The model under review builds one solid part; all positions refer to its coordinate system, in mm. A direction names the side the tool comes from. Coordinates: 2 decimals unless noted, no trailing zeros. Loops run counter-clockwise (first coordinate to the right, second up) from the corner with the lowest first, then second, coordinate; pieces in that order, holes last. Notation, with made-up numbers: M -36.75,1.5 L 18.25,1.5 A12 ccw 18.25,20.5 Z; hole C 70,22.25 d7. An arc over 180 degrees is marked long. Return JSON: item names as keys, results as strings.
```python
from build123d import *

# Parameters (mm, degrees)
SKETCH_1_W          = 220
SKETCH_1_H          = 180
EXTRUDE_1_DEPTH     = 395
SKETCH_17_W         = 46
SKETCH_17_H         = 45
CUT_EXTRUDE_2_DEPTH = 2
SKETCH_19_W         = 224
SKETCH_19_H         = 184
EXTRUDE_13_DEPTH    = 2
SKETCH_20_W         = 60
SKETCH_20_H         = 18
CUT_EXTRUDE_4_DEPTH = 65
SKETCH_21_W         = 144
SKETCH_21_H         = 332
CUT_EXTRUDE_5_DEPTH = 2
SKETCH_22_R         = 2.5
CUT_EXTRUDE_6_DEPTH = 10
SKETCH_23_R         = 11
SKETCH_23_R_2       = 2.25
SKETCH_23_R_3       = 1.5
CUT_EXTRUDE_7_DEPTH = 2
SKETCH_24_R         = 2
SKETCH_24_R_2       = 2.5
CUT_EXTRUDE_8_DEPTH = 3
CUT_EXTRUDE_9_DEPTH = 491.824815999
HOLE_WIZARD_M6_1_D  = 5


with BuildPart() as part:
    # 草图1 → 凸台-拉伸1 (new body)
    with BuildSketch(Plane(origin=(0, 0, 0), x_dir=(1, 0, 0), z_dir=(0, 1, 0))):
        Polygon((222, 2), (222, -182), (173, -182), (47, -182), (-2, -182), (-2, 2), align=None)
        with Locations((110, -90)):
            Rectangle(SKETCH_1_W, SKETCH_1_H, mode=Mode.SUBTRACT)
    extrude(amount=EXTRUDE_1_DEPTH)

    # 草图17 → 切除-拉伸2 (cut)
    with BuildSketch(Plane.XY.offset(182)):
        with Locations((23, 22.5)):
            Rectangle(SKETCH_17_W, SKETCH_17_H)
        with Locations((197, 22.5)):
            Rectangle(SKETCH_17_W, SKETCH_17_H)
    extrude(amount=-CUT_EXTRUDE_2_DEPTH, mode=Mode.SUBTRACT)

    # 草图19 → 凸台-拉伸13 (add)
    with BuildSketch(Plane(origin=(0, 395, 0), x_dir=(1, 0, 0), z_dir=(0, 1, 0))):
        with Locations((110, -90)):
            Rectangle(SKETCH_19_W, SKETCH_19_H)
    extrude(amount=EXTRUDE_13_DEPTH)

    # 草图20 → 切除-拉伸4 (cut)
    with BuildSketch(Plane.XY.offset(182)):
        with Locations((110, 390)):
            Rectangle(SKETCH_20_W, SKETCH_20_H)
    extrude(amount=-CUT_EXTRUDE_4_DEPTH, mode=Mode.SUBTRACT)

    # 草图21 → 切除-拉伸5 (cut)
    with BuildSketch(Plane(origin=(222, 0, 0), x_dir=(0, 0, -1), z_dir=(1, 0, 0))):
        with Locations((-90, 211)):
            Rectangle(SKETCH_21_W, SKETCH_21_H)
    extrude(amount=-CUT_EXTRUDE_5_DEPTH, mode=Mode.SUBTRACT)

    # 草图22 → 切除-拉伸6 (cut)
    with BuildSketch(Plane(origin=(0, 397, 0), x_dir=(1, 0, 0), z_dir=(0, 1, 0))):
        with Locations(Location((77.7, -25.2, 0), (0, 0, 270))):
            Circle(SKETCH_22_R)
        with Locations(Location((77.7, -89.8, 0), (0, 0, 270))):
            Circle(SKETCH_22_R)
        with Locations(Location((142.3, -89.8, 0), (0, 0, 270))):
            Circle(SKETCH_22_R)
        with Locations(Location((142.3, -25.2, 0), (0, 0, 270))):
            Circle(SKETCH_22_R)
        Polygon((74, -57.5), (74, -81.5), (146, -81.5), (146, -33.5), (74, -33.5), align=None)
    extrude(amount=-CUT_EXTRUDE_6_DEPTH, mode=Mode.SUBTRACT)

    # 草图23 → 切除-拉伸7 (cut)
    with BuildSketch(Plane(origin=(0, 0, -2), x_dir=(-1, 0, 0), z_dir=(0, 0, -1))):
        with Locations((-183.5, 217.109875683)):
            Circle(SKETCH_23_R)
        with Locations((-203.5, 88.459875683)):
            Circle(SKETCH_23_R_2)
        with Locations((-163.5, 88.459875683)):
            Circle(SKETCH_23_R_2)
        with Locations((-183.5, 180.109875683)):
            Circle(SKETCH_23_R)
        with Locations((-183.5, 254.109875683)):
            Circle(SKETCH_23_R)
        with Locations((-171.8, 147.859875683)):
            Circle(SKETCH_23_R_3)
        with Locations(Location((-195.2, 147.859875683, 0), (0, 0, 180))):
            Circle(SKETCH_23_R_3)
        Polygon((-183.5, 111.959875683), (-197.25, 111.959875683), (-197.25, 64.959875683), (-169.75, 64.959875683), (-169.75, 111.959875683), align=None)
        Polygon((-183.5, 151.609875683), (-175, 151.609875683), (-175.5, 143.109875683), (-183.5, 143.109875683), (-191.5, 143.109875683), (-192, 151.609875683), align=None)
    extrude(amount=-CUT_EXTRUDE_7_DEPTH, mode=Mode.SUBTRACT)

    # 草图24 → 切除-拉伸8 (cut)
    with BuildSketch(Plane(origin=(222, 0, 0), x_dir=(0, 0, -1), z_dir=(1, 0, 0))):
        with Locations((-169.5, 362)):
            Circle(SKETCH_24_R)
        with Locations((-169.5, 347)):
            Circle(SKETCH_24_R)
        with Locations(Location((-169.5, 75, 0), (0, 0, 180))):
            Circle(SKETCH_24_R)
        with Locations(Location((-169.5, 60, 0), (0, 0, 180))):
            Circle(SKETCH_24_R)
        with Locations((-10.5, 211)):
            Circle(SKETCH_24_R_2)
    extrude(amount=-CUT_EXTRUDE_8_DEPTH, mode=Mode.SUBTRACT)

    # 草图25 → 切除-拉伸9 (cut, through all)
    with BuildSketch(Plane(origin=(222, 0, 0), x_dir=(0, 0, -1), z_dir=(1, 0, 0))):
        with BuildLine():
            Line((-15, 16), (-30, 16))
            ThreePointArc((-30, 16), (-34, 20), (-30, 24))
            Line((-30, 24), (-15, 24))
            ThreePointArc((-15, 24), (-11, 20), (-15, 16))
        make_face()
    extrude(amount=-CUT_EXTRUDE_9_DEPTH, mode=Mode.SUBTRACT)

    # M6 螺纹孔1 (through all)
    with Locations(Plane(origin=(0, 397, 0), x_dir=(1, 0, 0), z_dir=(0, 1, 0))):
        with Locations((186, -90), (34, -90)):
            Hole(HOLE_WIZARD_M6_1_D / 2)


solid = part.part
```
1. The part is to be moulded in two halves that separate along Y. For faces 1 (the face through (108, 395, 89)), 2 (the face through (194.49, 217.59, -1.01)), 3 (the face through (108, 196, 182)), say which applies: released by +Y, released by -Y, zero draft, split by the parting line, or undercut.
Check values:
{"face 1": "released by -Y", "face 2": "undercut", "face 3": "zero draft"}
2. Add section A-A on z = 152. Give the boundary of the cut face in (x, y), plus the area to 3 significant figures.
Check values:
{"outline": "M -2,0 L 0,0 L 0,395 L 80,395 L 80,397 L -2,397 Z; M 140,395 L 220,395 L 220,377 L 222,377 L 222,397 L 140,397 Z; M 220,0 L 222,0 L 222,45 L 220,45 Z", "area": "1,240 mm²"}
3. To check wall thickness, follow line 1 (Z direction, x = 142, y = 396); line 2 (Y direction, x = 220.5, z = 169.5); line 3 (Z direction, x = 18.5, y = 163). State the ranges of each line that lie inside material, in increasing order.
Check values:
{"line 1": "-2 to 22.72, 27.68 to 33.5, 81.5 to 87.32, 92.28 to 182", "line 2": "0 to 58, 62 to 73, 77 to 345, 349 to 360, 364 to 397", "line 3": "-2 to 0, 180 to 182"}
4. Add section D-D on y = 20. Give the boundary of the cut face in (x, z).
Check values:
{"outline": "M -2,-2 L 222,-2 L 222,11 L 220,11 L 220,0 L 0,0 L 0,11 L -2,11 Z; M -2,34 L 0,34 L 0,182 L -2,182 Z; M 46,180 L 174,180 L 174,182 L 46,182 Z; M 220,34 L 222,34 L 222,182 L 220,182 Z"}
5. Add section C-C on z = 105.5. Give the boundary of the cut face in (x, y).
Check values:
{"outline": "M -2,0 L 0,0 L 0,395 L 220,395 L 220,377 L 222,377 L 222,397 L -2,397 Z; M 220,0 L 222,0 L 222,45 L 220,45 Z"}
6. Machinability: for faces 4 (the face through (108, 196, -2)), 5 (the face through (108, 195, 180)), 6 (the face through (-2, 196, 91)), 7 (the face through (80, 395.5, 156.9)), 8 (the face through (194.49, 180.59, -1.01)), which of the approach directions +Z, -Z, +X, -X, +Y, -Y give a long, thin tool a straight path to every point of the face, cutting with its end or side? Answer none if there is none.
Check values:
{"face 4": "-Z, +X, -X, +Y, -Y", "face 5": "-Y", "face 6": "+Z, -Z, -X, +Y, -Y", "face 7": "+Z, +Y", "face 8": "-Z"}
7. Insertion check: pin 1 Ø12 at (x, z) = (181.5, 32.5) entering from -Y; pin 2 Ø3 at (y, z) = (354.5, 152.5) entering from +X. Each pin has a flat end and moves straight along its axis. Give the tip position at first contact, or say it passes through.
Check values:
{"pin 1": "y = 395", "pin 2": "x = 0"}
8. Add section B-B on y = 105.5. Give the boundary of the cut face in (x, z), plus the area to 3 significant figures.
Check values:
{"outline": "M -2,-2 L 169.75,-2 L 169.75,0 L 0,0 L 0,180 L 220,180 L 220,162 L 222,162 L 222,182 L -2,182 Z; M 197.25,-2 L 222,-2 L 222,18 L 220,18 L 220,0 L 197.25,0 Z", "area": "1,270 mm²"}
